from build123d import *
from build123d.topology import SkipClean

# Parameters (mm, degrees)
SKETCH2_R               = 5.25
BOSS_EXTRUDE1_DEPTH     = 14
CUT_EXTRUDE1_DEPTH      = 1
CUT_EXTRUDE2_DEPTH      = 1
BOSS_EXTRUDE2_DEPTH     = 9
BOSS_EXTRUDE3_DEPTH     = 9.5
FILLET1_R               = 1
FILLET1_OF_MIRROR1_R    = 1
CUT_EXTRUDE3_DEPTH      = 57.347138959
CUT_EXTRUDE3_DEPTH_BACK = 57.347138959
BOSS_EXTRUDE4_DEPTH     = 1.5


with BuildPart() as part:
    # Sketch2 → Boss-Extrude1 (new body)
    with BuildSketch(Plane(origin=(0, 0, 0), x_dir=(0, 0, -1), z_dir=(1, 0, 0))):
        with BuildLine():
            ThreePointArc((0, 0), (9, 9), (0, 18))
            Line((0, 18), (-4.055355956, 18))
            Line((-4.055355956, 18), (-14.1, 8.3))
            Line((-14.1, 8.3), (-22.975773924, 5.754912782))
            ThreePointArc((-22.975773924, 5.754912782), (-23.743647767, 6.106105344), (-24.576075178, 6.24763647))
            Line((-24.576075178, 6.24763647), (-45.007968978, 23.392031022))
            Line((-45.007968978, 23.392031022), (-47.2, 21.2))
            Line((-47.2, 21.2), (-27.661634154, 1.661634154))
            ThreePointArc((-27.661634154, 1.661634154), (-25.892761453, -0.023213541), (-23.45, 0))
            Line((-23.45, 0), (0, 0))
        make_face()
        with Locations((0, 9)):
            Circle(SKETCH2_R, mode=Mode.SUBTRACT)
    boss_extrude1 = extrude(amount=-BOSS_EXTRUDE1_DEPTH)

    # Sketch2_5 → Cut-Extrude1 (cut)
    with BuildSketch(Plane(origin=(0, 0, 0), x_dir=(0, 0, -1), z_dir=(1, 0, 0))):
        with BuildLine():
            Line((-29.259155366, 3.259155366), (-27.661634154, 1.661634154))
            ThreePointArc((-27.661634154, 1.661634154), (-27.396479719, 4.814248364), (-24.576075178, 6.24763647))
            Line((-24.576075178, 6.24763647), (-25.89413767, 7.35362222))
            ThreePointArc((-25.89413767, 7.35362222), (-25.722467199, 6.887608312), (-26.037233654, 6.503470587))
            ThreePointArc((-26.037233654, 6.503470587), (-27.626659815, 5.344602808), (-28.410825273, 3.540625374))
            ThreePointArc((-28.410825273, 3.540625374), (-28.748146118, 3.138148273), (-29.259155366, 3.259155366))
        make_face()
    cut_extrude1 = extrude(amount=-CUT_EXTRUDE1_DEPTH, mode=Mode.SUBTRACT)

    # Sketch2_6 → Cut-Extrude2 (cut)
    with SkipClean():  # the faces are left unmerged after this step: merging them gives an invalid solid
        with BuildSketch(Plane(origin=(0, 0, 0), x_dir=(0, 0, -1), z_dir=(1, 0, 0))):
            with BuildLine():
                Line((-23.45, 0), (-21.263068229, 0))
                ThreePointArc((-21.263068229, 0), (-21.708634623, 0.273128697), (-21.667413143, 0.794117647))
                ThreePointArc((-21.667413143, 0.794117647), (-20.951415597, 3.103028999), (-21.793156226, 5.369126268))
                ThreePointArc((-21.793156226, 5.369126268), (-21.882671913, 5.8346109), (-21.543395734, 6.165640619))
                Line((-21.543395734, 6.165640619), (-22.975773924, 5.754912782))
                ThreePointArc((-22.975773924, 5.754912782), (-21.856917628, 4.574605546), (-21.45, 3))
                ThreePointArc((-21.45, 3), (-21.995836543, 1.197224362), (-23.45, 0))
            make_face()
        cut_extrude2 = extrude(amount=-CUT_EXTRUDE2_DEPTH, mode=Mode.SUBTRACT)

    # Sketch3 → Boss-Extrude2 (add)
    with SkipClean():  # the faces are left unmerged after this step: merging them gives an invalid solid
        with BuildSketch(Plane.ZY.offset(14)):
            with BuildLine():
                ThreePointArc((23.45, 0), (21.46097847, 2.733092659), (22.975773924, 5.754912782))
                Line((22.975773924, 5.754912782), (14.1, 8.3))
                Line((14.1, 8.3), (11.259590113, 9.114474429))
                ThreePointArc((11.259590113, 9.114474429), (10.41329932, 8.974403731), (9.986911251, 8.230077781))
                ThreePointArc((9.986911251, 8.230077781), (9.041706899, 4.689696888), (6.886416056, 1.726180477))
                ThreePointArc((6.886416056, 1.726180477), (6.644893676, 0.629986809), (7.573920177, 0))
                Line((7.573920177, 0), (23.45, 0))
            make_face()
            with BuildLine():
                ThreePointArc((27.95, 3), (26.953857175, 5.341501193), (24.576075178, 6.24763647))
                ThreePointArc((24.576075178, 6.24763647), (23.743647767, 6.106105344), (22.975773924, 5.754912782))
                ThreePointArc((22.975773924, 5.754912782), (21.46097847, 2.733092659), (23.45, 0))
                ThreePointArc((23.45, 0), (25.892761453, -0.023213541), (27.661634154, 1.661634154))
                ThreePointArc((27.661634154, 1.661634154), (27.877090729, 2.315460374), (27.95, 3))
            make_face()
            with BuildLine():
                Line((47.2, 21.2), (45.007968978, 23.392031022))
                Line((45.007968978, 23.392031022), (24.576075178, 6.24763647))
                ThreePointArc((24.576075178, 6.24763647), (26.953857175, 5.341501193), (27.95, 3))
                ThreePointArc((27.95, 3), (27.877090729, 2.315460374), (27.661634154, 1.661634154))
                Line((27.661634154, 1.661634154), (47.2, 21.2))
            make_face()
        boss_extrude2 = extrude(amount=BOSS_EXTRUDE2_DEPTH)

    # Sketch3_3 → Boss-Extrude3 (add)
    with SkipClean():  # the faces are left unmerged after this step: merging them gives an invalid solid
        with BuildSketch(Plane.ZY.offset(14)):
            with BuildLine():
                ThreePointArc((27.95, 3), (26.953857175, 5.341501193), (24.576075178, 6.24763647))
                ThreePointArc((24.576075178, 6.24763647), (23.743647767, 6.106105344), (22.975773924, 5.754912782))
                ThreePointArc((22.975773924, 5.754912782), (21.46097847, 2.733092659), (23.45, 0))
                ThreePointArc((23.45, 0), (25.892761453, -0.023213541), (27.661634154, 1.661634154))
                ThreePointArc((27.661634154, 1.661634154), (27.877090729, 2.315460374), (27.95, 3))
            make_face()
        boss_extrude3 = extrude(amount=BOSS_EXTRUDE3_DEPTH)

    # Fillet1
    fillet1_edges = [part.edges().sort_by_distance(p)[0] for p in [
        (-7, 18, 4.055355956),
    ]]
    fillet(fillet1_edges, radius=FILLET1_R)

    # Mirror1: Boss-Extrude1, Cut-Extrude1, Cut-Extrude2, Boss-Extrude2, Boss-Extrude3 across plane
    with SkipClean():  # the faces are left unmerged after this step: merging them gives an invalid solid
        add(boss_extrude1.mirror(Plane(origin=(0, 0, 0), x_dir=(0, 0, 1), z_dir=(1, 0, 0))))
        add(cut_extrude1.mirror(Plane(origin=(0, 0, 0), x_dir=(0, 0, 1), z_dir=(1, 0, 0))), mode=Mode.SUBTRACT)
        add(cut_extrude2.mirror(Plane(origin=(0, 0, 0), x_dir=(0, 0, 1), z_dir=(1, 0, 0))), mode=Mode.SUBTRACT)
        add(boss_extrude2.mirror(Plane(origin=(0, 0, 0), x_dir=(0, 0, 1), z_dir=(1, 0, 0))))
        add(boss_extrude3.mirror(Plane(origin=(0, 0, 0), x_dir=(0, 0, 1), z_dir=(1, 0, 0))))

    # Fillet1 of Mirror1
    fillet1_of_mirror1_edges = [part.edges().sort_by_distance(p)[0] for p in [
        (7, 18, 4.055355956),
    ]]
    fillet(fillet1_of_mirror1_edges, radius=FILLET1_OF_MIRROR1_R)

    # Sketch4 → Cut-Extrude3 (cut, two sides: drawn at the far end of the back side and taken through both)
    with SkipClean():  # the faces are left unmerged after this step: merging them gives an invalid solid
        with BuildSketch(Plane(origin=(0, -8.435091108, 7.077881838), x_dir=(1, 0, 0), z_dir=(0, 0.7660444431189767, -0.6427876096865409)).offset(-CUT_EXTRUDE3_DEPTH_BACK)):
            Polygon((0, 0), (0, -53.228637451), (-37.92308493, -53.228637451), (-37.92308493, 7.135530727), (0, 7.135530727), align=None)
        extrude(amount=CUT_EXTRUDE3_DEPTH + CUT_EXTRUDE3_DEPTH_BACK, mode=Mode.SUBTRACT)

    # Sketch7 → Boss-Extrude4 (add)
    with SkipClean():  # the faces are left unmerged after this step: merging them gives an invalid solid
        with BuildSketch(Plane(origin=(23, 0, 0), x_dir=(0, 0, -1), z_dir=(1, 0, 0))):
            with BuildLine():
                ThreePointArc((-27.661634154, 1.661634154), (-27.396479719, 4.814248364), (-24.576075178, 6.24763647))
                Line((-24.576075178, 6.24763647), (-45.007968978, 23.392031022))
                Line((-45.007968978, 23.392031022), (-47.2, 21.2))
                Line((-47.2, 21.2), (-27.661634154, 1.661634154))
            make_face()
            with BuildLine():
                ThreePointArc((-21.45, 3), (-21.856917628, 4.574605546), (-22.975773924, 5.754912782))
                ThreePointArc((-22.975773924, 5.754912782), (-23.743647767, 6.106105344), (-24.576075178, 6.24763647))
                ThreePointArc((-24.576075178, 6.24763647), (-27.396479719, 4.814248364), (-27.661634154, 1.661634154))
                ThreePointArc((-27.661634154, 1.661634154), (-25.892761453, -0.023213541), (-23.45, 0))
                ThreePointArc((-23.45, 0), (-21.995836543, 1.197224362), (-21.45, 3))
            make_face()
            with BuildLine():
                Line((-11.259590113, 9.114474429), (-22.975773924, 5.754912782))
                ThreePointArc((-22.975773924, 5.754912782), (-21.856917628, 4.574605546), (-21.45, 3))
                ThreePointArc((-21.45, 3), (-21.995836543, 1.197224362), (-23.45, 0))
                Line((-23.45, 0), (-7.573920177, 0))
                ThreePointArc((-7.573920177, 0), (-8.502946677, 1.370013191), (-6.886416056, 1.726180477))
                ThreePointArc((-6.886416056, 1.726180477), (-9.041706899, 4.689696888), (-9.986911251, 8.230077781))
                ThreePointArc((-9.986911251, 8.230077781), (-9.984692654, 8.191673714), (-9.983952757, 8.153212733))
                ThreePointArc((-9.983952757, 8.153212733), (-11.58576778, 7.354577223), (-11.259590113, 9.114474429))
            make_face()
            with BuildLine():
                ThreePointArc((-9.986911251, 8.230077781), (-10.41329932, 8.974403731), (-11.259590113, 9.114474429))
                ThreePointArc((-11.259590113, 9.114474429), (-11.58576778, 7.354577223), (-9.983952757, 8.153212733))
                ThreePointArc((-9.983952757, 8.153212733), (-9.984692654, 8.191673714), (-9.986911251, 8.230077781))
            make_face()
            with BuildLine():
                ThreePointArc((-6.573920177, 1), (-6.655360402, 1.395282102), (-6.886416056, 1.726180477))
                ThreePointArc((-6.886416056, 1.726180477), (-8.502946677, 1.370013191), (-7.573920177, 0))
                ThreePointArc((-7.573920177, 0), (-6.866813396, 0.292893219), (-6.573920177, 1))
            make_face()
        extrude(amount=BOSS_EXTRUDE4_DEPTH)

    # Mirror14: part across plane


with BuildPart() as part_1:
    with SkipClean():  # the faces are left unmerged after this step: merging them gives an invalid solid
        add(part.part)
        add(part.part.mirror(Plane(origin=(24.5, 0, 0), x_dir=(0, 0, 1), z_dir=(1, 0, 0))))


solid = part_1.part
Could you check a few things on this model? Use its own coordinates, in mm. A direction names the side the tool comes from. Give positions to 0.01 mm unless a question says otherwise; leave off trailing zeros. Order: outer loops, then holes, each group sorted by start corner. A loop starts at its lowest first (then second) coordinate and runs counter-clockwise, first axis right, second up. Notation, with made-up numbers: (22.5, 46.25) -> (55.5, 46.25) arc R13 ccw to (55.5, 56.25) -> close; hole circle Ø10 at (58.25, -34.5). An arc over 180 degrees is marked (long way). Answer in a Markdown table with one row per item. Add a question column.
Item 1: Imagine slicing it at A-A (x = 38). List the corners of the cut face in (y, z) for me.
Item 2: Imagine slicing it at B-B (y = 13.5). List the corners of the cut face in (x, z) for me.
Item 3: We'd pull the mould along Y, two halves only. Please class faces 1 (the flat face through (1, 3.1, 21.3)), 2 (the cylindrical face through (42, 9, -9)), 3 (the flat face through (49, 3, 25)), 4 (the flat face through (24.84, 14.7, 34.65)): pulls with the +Y half, pulls with the -Y half, needs draft (parallel to the pull), parting line crosses it, or undercut.
Item 4: I'm going to push flat-ended pins straight in: P1, Ø5, axis at x = 8, z = 10.5, coming from the +Y side; P2, Ø4, axis at x = 5.5, z = 2.5, coming from the +Y side; P3, Ø5, axis at x = 8.5, y = 2.5, coming from the +Z side. Where does each tip first touch, or does it pass through?
Item 5: For faces 5 (the flat face through (6.9, 13.08, 9.15)), 6 (the flat face through (7, 18, 2)), 7 (the flat face through (1, 5.2, 27.3)), 8 (the flat face through (0, 3, 25)), 9 (the flat face through (48, 5.2, 27.3)), which set-ups out of +Z, -Z, +X, -X, +Y, -Y let a thin tool reach every point of the face, with its end or its side?
Item 6: Imagine slicing it at C-C (z = 2.5). List the corners of the cut face in (x, y) for me, and give its area (3 significant figures).
Item 7: Please list where these lines run through material, in increasing order: probe 1 along X at (y, z) = (2.75, 7); probe 2 along Z at (x, y) = (10.25, 9); probe 3 along Z at (x, y) = (12, 11.25).
Item 8: Imagine slicing it at D-D (x = 29). List the corners of the cut face in (y, z) for me, and give its area (3 significant figures).
Result:
| question | item | result |
|---|---|---|
| 1 | outline | (0, 0) arc R9 ccw to (18, 0) -> (18, 3.65) arc R1 ccw to (17.72, 4.35) -> (8.3, 14.1) -> (5.75, 22.98) arc R3.25 ccw to (6.25, 24.58) -> (23.39, 45.01) -> (21.2, 47.2) -> (1.66, 27.66) arc R3.25 ccw to (0, 23.45) -> close; hole circle Ø10.5 at (9, 0) |
| 2 | outline | (0, -7.79) -> (14, -7.79) -> (14, -2.7) -> (0, -2.7) -> close; (0, 2.7) -> (14, 2.7) -> (14, 8.72) -> (0, 8.72) -> close; (0, 33.22) -> (49, 33.22) -> (49, 39.5) -> (0, 39.5) -> close; (35, -7.79) -> (49, -7.79) -> (49, -2.7) -> (35, -2.7) -> close; (35, 2.7) -> (49, 2.7) -> (49, 8.72) -> (35, 8.72) -> close |
| 3 | face 1 | undercut |
| 3 | face 2 | parting line crosses it |
| 3 | face 3 | needs draft |
| 3 | face 4 | pulls with the +Y half |
| 4 | P1 | y = 14.19 |
| 4 | P2 | y = 18 |
| 4 | P3 | z = 31 |
| 5 | face 5 | +X, -X, +Y |
| 5 | face 6 | -Z, +X, -X, +Y |
| 5 | face 7 | -X |
| 5 | face 8 | +Z, -Z, -X, +Y, -Y |
| 5 | face 9 | +X |
| 6 | outline | (0, 0) -> (14, 0) -> (14, 4.38) -> (0, 4.38) -> close; (0, 13.62) -> (14, 13.62) -> (14, 18) -> (0, 18) -> close; (35, 0) -> (49, 0) -> (49, 4.38) -> (35, 4.38) -> close; (35, 13.62) -> (49, 13.62) -> (49, 18) -> (35, 18) -> close |
| 6 | area | 245 mm2 |
| 7 | probe 1 | 0 to 14, 35 to 49 |
| 7 | probe 2 | -9 to -5.25, 5.25 to 13.38, 27.86 to 35 |
| 7 | probe 3 | -8.71 to -4.74, 4.74 to 11.05, 30.54 to 37.25 |
| 8 | outline | (0, 7.57) arc R1 ccw to (1.73, 6.89) arc R10.02 cw to (8.23, 9.99) arc R1 ccw to (9.11, 11.26) -> (5.75, 22.98) arc R3.25 ccw to (6.25, 24.58) -> (23.39, 45.01) -> (21.2, 47.2) -> (1.66, 27.66) arc R3.25 ccw to (0, 23.45) -> close |
| 8 | area | 248 mm2 |
